The model under review builds one solid part; all positions refer to its coordinate system, in mm. Coordinates: 2 decimals unless noted, no trailing zeros. Loops run counter-clockwise (first coordinate to the right, second up) from the corner with the lowest first, then second, coordinate; pieces in that order, holes last. Notation, with made-up numbers: M 78.25,39.25 L 85.25,39.25 A21 ccw 85.25,73.25 Z; hole C -39.5,-36 d5. An arc over 180 degrees is marked long. One line per item, written item: value.
Autodesk Inventor part; units mm, degrees
ref_plane "YZ Plane" through (0, 0, 0) normal (1, 0, 0) x (0, 1, 0)
ref_plane "XZ Plane" through (0, 0, 0) normal (0, 1, 0) x (-1, 0, 0)
ref_plane "XY Plane" through (0, 0, 0) normal (0, 0, 1) x (1, 0, 0)
sketch "Boceto1" plane through (0, 0, 0) normal (0, 1, 0) x (-1, 0, 0)
  line L0 (4, 5) -> (4, 18.57)
  line L1 (4, 18.57) -> (-16, 18.57)
  line L2 (-16, 18.57) -> (-16, -18.57)
  line L3 (-16, -18.57) -> (4, -18.57)
  line L4 (4, -18.57) -> (4, -5)
  line L5 (0, -5) -> (0, -11)
  line L6 (0, 5) -> (0, 11)
  line L7 (0, -11) -> (-12, -11)
  line L8 (0, 11) -> (-12, 11)
  circle A0 centre (0, 11) radius 2
  circle A1 centre (0, -11) radius 2
  circle A2 centre (-12, -11) radius 2
  circle A3 centre (-12, 11) radius 2
  line L9 (4, -5) -> (4, 5)
  point P0 (0, 0)
  dimension "d0" = 5
  dimension "d1" = 4
  dimension "d2" = 13.57
  dimension "d3" = 20
  dimension "d4" = 37.14
  dimension "d5" = 20
  dimension "d6" = 13.57
  dimension "d7" = 4
  dimension "d8" = 6
  dimension "d9" = 6
  dimension "d11" = 12
  dimension "d12" = 12
  dimension "d13" = 4
  dimension "d14" = 4
  dimension "d15" = 4
  dimension "d16" = 4
extrude "Extrusión1" add sketch "Boceto1" along normal blind 5
equation "\"Radio_pliegue\" = Grosor"
equation "\"Anchura_desahogo_plegado\" = Grosor"
equation "\"Profundidad_desahogo_plegado\" = 0.5 * Grosor"
equation "\"Tamaño_destalonado\" = 4 * Grosor"
equation "\"Remanente_mínimo\" = 2 * Grosor"
equation "\"Radiodetransición\" = Radio_pliegue"
equation "\"Tamaño_de_radio_de_Jacobi\" = Radio_pliegue"
equation "\"TamañoSeparación\" = Grosor"
properties part number "Sujetador"
(1) Draft analysis for pull direction Z (two halves, no side actions). For faces 1 (the face through (16, 2, 0)), 2 (the face through (6, 2, -18.57)), 3 (the face through (13.474, 2.465, 9.648)), state which applies: pulls with the +Z half, pulls with the -Z half, needs draft (parallel to the pull), parting line crosses it, or undercut.
Checks:
face 1: needs draft
face 2: pulls with the -Z half
face 3: undercut
(2) Add section A-A on z = 11. State the section outline as (x, y) points, then the cut area to 3 significant figures.
Checks:
outline: M -4,0 L -2,0 L -2,5 L -4,5 Z; M 2,0 L 10,0 L 10,5 L 2,5 Z; M 14,0 L 16,0 L 16,5 L 14,5 Z
area: 60.0 mm^2
(3) Add section B-B on x = 12. State the section outline as (y, z) points.
Checks:
outline: M 0,-18.57 L 5,-18.57 L 5,-13 L 0,-13 Z; M 0,-9 L 5,-9 L 5,9 L 0,9 Z; M 0,13 L 5,13 L 5,18.57 L 0,18.57 Z
(4) Add section C-C on y = 4. State the section outline as (x, z) points.
Checks:
outline: M -4,-18.57 L 16,-18.57 L 16,18.57 L -4,18.57 Z; hole C 0,-11 d4; hole C 0,11 d4; hole C 12,-11 d4; hole C 12,11 d4
(5) To check wall thickness, follow L1, parallel to Z at x = 0, y = 1; L2, parallel to Z at x = 13.5, y = 4.65; L3, parallel to X at y = 1.6, z = 9.5. State the ranges of each line that lie inside material, in increasing order. Write a range as [from, to].
Checks:
L1: [-18.57, -13], [-9, 9], [13, 18.57]
L2: [-18.57, -12.32], [-9.68, 9.68], [12.32, 18.57]
L3: [-4, -1.32], [1.32, 10.68], [13.32, 16]
(6) Insertion check: pin 1 Ø3.5 at (x, z) = (0, 11) entering from +Y. The pin has a flat end and moves straight along its axis. Give the tip position at first contact, or say it passes through.
Checks:
pin 1: through
